Read the model definition and answer for the solid it produces. Units are mm, in the model's axes. Round coordinates to 2 decimals unless told otherwise and drop trailing zeros. Write each loop counter-clockwise with the first axis right and the second up, starting at its lowest first coordinate (ties: lowest second). Pieces come first, ordered by that corner, then holes.
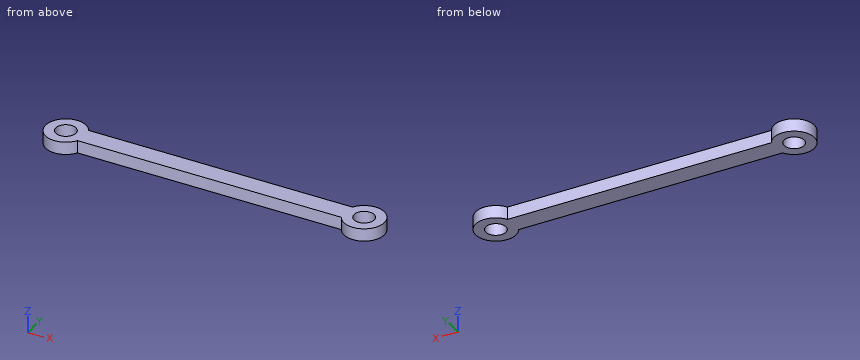
from build123d import *

# Parameters (mm, degrees)
SKETCH1_R           = 5.08
SKETCH1_W           = 76.2
SKETCH1_H           = 5.08
BOSS_EXTRUDE1_DEPTH = 3.175
SKETCH2_R           = 2.54
CUT_EXTRUDE1_DEPTH  = 82.698123754


with BuildPart() as part:
    # Sketch1 → Boss-Extrude1 (new body)
    with BuildSketch(Plane.XY):
        with Locations((0, 2.54)):
            Circle(SKETCH1_R)
        with Locations((76.2, 2.54)):
            Circle(SKETCH1_R)
        with Locations((38.1, 2.54)):
            Rectangle(SKETCH1_W, SKETCH1_H)
    extrude(amount=BOSS_EXTRUDE1_DEPTH)

    # Sketch2 → Cut-Extrude1 (cut, through all)
    with BuildSketch(Plane.XY.offset(3.175)):
        with Locations((0, 2.54)):
            Circle(SKETCH2_R)
        with Locations((76.2, 2.54)):
            Circle(SKETCH2_R)
    extrude(amount=-CUT_EXTRUDE1_DEPTH, mode=Mode.SUBTRACT)


solid = part.part
Q1. A flat-ended cylindrical pin translates along its axis: pin 1 Ø1 at (x, y) = (17.5, 4) entering from -Z. Find the tip coordinate at first contact, or state that the pin passes through.
Verdict:
pin 1: stops at z = 0
Q2. Section C-C (z = 2.6) is taken. Determine the outline of the cut face in (x, y), then the cut area to 3 significant figures.
Verdict:
outline: (4.4, 0) - (71.8, 0) arc R5.08 ccw (long way) to (71.8, 5.08) - (4.4, 5.08) arc R5.08 ccw (long way) to start; hole circle Ø5.08 at (0, 2.54); hole circle Ø5.08 at (76.2, 2.54)
area: 459 mm2
Q3. Section A-A (x = 76.2) is taken. Determine the outline of the cut face in (y, z) (3 decimals).
Verdict:
outline: (-2.54, 0) - (0, 0) - (0, 3.175) - (-2.54, 3.175) - close; (5.08, 0) - (7.62, 0) - (7.62, 3.175) - (5.08, 3.175) - close
Q4. Section B-B (y = 2.54) is taken. Determine the outline of the cut face in (x, z) (3 decimals), then the cut area to 3 significant figures.
Verdict:
outline: (-5.08, 0) - (-2.54, 0) - (-2.54, 3.175) - (-5.08, 3.175) - close; (2.54, 0) - (73.66, 0) - (73.66, 3.175) - (2.54, 3.175) - close; (78.74, 0) - (81.28, 0) - (81.28, 3.175) - (78.74, 3.175) - close
area: 242 mm2
Q5. Section D-D (y = 6) is taken. Determine the outline of the cut face in (x, z) (3 decimals), then the cut area to 3 significant figures.
Verdict:
outline: (-3.72, 0) - (3.72, 0) - (3.72, 3.175) - (-3.72, 3.175) - close; (72.48, 0) - (79.92, 0) - (79.92, 3.175) - (72.48, 3.175) - close
area: 47.2 mm2
Q6. Straight lines are drawn through the part: probe 1 along X at (y, z) = (0.25, 0.95); probe 2 along X at (y, z) = (3.25, 1.6); probe 3 along Y at (x, z) = (76.2, 1.05). For each, find the intervals that lie inside material, in ascending order.
Verdict:
probe 1: x = -4.53 to -1.1, 1.1 to 75.1, 77.3 to 80.73
probe 2: x = -5.03 to -2.44, 2.44 to 73.76, 78.64 to 81.23
probe 3: y = -2.54 to 0, 5.08 to 7.62
